Read the model definition and answer for the solid it produces. Units are mm, in the model's axes. Give positions to 0.01 mm unless a question says otherwise; leave off trailing zeros. Write each loop counter-clockwise with the first axis right and the second up, starting at its lowest first coordinate (ties: lowest second). Pieces come first, ordered by that corner, then holes. Notation, with made-up numbers: (-30, -32.75) -> (18, -32.75) arc R21 cw to (18, -15.75) -> close; hole circle Ø9 at (-38, 32.5). An arc over 180 degrees is marked (long way). Use a Markdown table: item, result.
from build123d import *

# Parameters (mm, degrees)
CROQUIS1_R              = 2
CROQUIS1_R_2            = 2.1
SALIENTE_EXTRUIR1_DEPTH = 2


with BuildPart() as part:
    # Croquis1 → Saliente-Extruir1 (new body)
    with BuildSketch(Plane(origin=(0, 0, 0), x_dir=(1, 0, 0), z_dir=(0, 1, 0))):
        with BuildLine():
            Line((-8, 5.5), (8, 5.5))
            ThreePointArc((8, 5.5), (11.5, 0), (8, -5.5))
            Line((8, -5.5), (-8, -5.5))
            ThreePointArc((-8, -5.5), (-11.5, 0), (-8, 5.5))
        make_face()
        with Locations(Location((8, 0, 0), (0, 0, 270))):
            Circle(CROQUIS1_R, mode=Mode.SUBTRACT)
        with Locations(Location((0, 0, 0), (0, 0, 270))):
            Circle(CROQUIS1_R_2, mode=Mode.SUBTRACT)
        with Locations(Location((-8, 0, 0), (0, 0, 270))):
            Circle(CROQUIS1_R, mode=Mode.SUBTRACT)
    extrude(amount=SALIENTE_EXTRUIR1_DEPTH)


solid = part.part
Item 1: Straight lines are drawn through the part: line 1 along X through (y, z) = (1.75, -1.25); line 2 along Z through (x, y) = (-0.5, 0.9); line 3 along Z through (x, y) = (-9, 0.6). For each, find the intervals that lie inside material, in ascending order. Write a range as [from, to].
Return value:
| item | result |
|---|---|
| line 1 | [-11.37, -9.56], [-6.44, -1.69], [1.69, 6.44], [9.56, 11.37] |
| line 2 | [-5.5, -2.04], [2.04, 5.5] |
| line 3 | [-4.91, -1.73], [1.73, 4.91] |
Item 2: A cutting plane is placed at C-C (z = -1). Give the vertices of the cut face in (x, y), then the cut area to 3 significant figures.
Return value:
| item | result |
|---|---|
| outline | (-11.42, 0) -> (-9.73, 0) -> (-9.73, 2) -> (-11.42, 2) -> close; (-6.27, 0) -> (-1.85, 0) -> (-1.85, 2) -> (-6.27, 2) -> close; (1.85, 0) -> (6.27, 0) -> (6.27, 2) -> (1.85, 2) -> close; (9.73, 0) -> (11.42, 0) -> (11.42, 2) -> (9.73, 2) -> close |
| area | 24.4 mm^2 |
Item 3: A cutting plane is placed at D-D (x = 7). Give the vertices of the cut face in (y, z).
Return value:
| item | result |
|---|---|
| outline | (0, -5.5) -> (2, -5.5) -> (2, -1.73) -> (0, -1.73) -> close; (0, 1.73) -> (2, 1.73) -> (2, 5.5) -> (0, 5.5) -> close |
Item 4: A cutting plane is placed at B-B (x = 0). Give the vertices of the cut face in (y, z).
Return value:
| item | result |
|---|---|
| outline | (0, -5.5) -> (2, -5.5) -> (2, -2.1) -> (0, -2.1) -> close; (0, 2.1) -> (2, 2.1) -> (2, 5.5) -> (0, 5.5) -> close |
Item 5: A cutting plane is placed at A-A (y = 1.2). Give the vertices of the cut face in (x, z).
Return value:
| item | result |
|---|---|
| outline | (-8, -5.5) -> (8, -5.5) arc R6.07 ccw to (8, 5.5) -> (-8, 5.5) arc R6.07 ccw to start; hole circle Ø4 at (-8, 0); hole circle Ø4.2 at (0, 0); hole circle Ø4 at (8, 0) |
Item 6: For a pull along X with two mould halves and no side action, classify faces 1 (the face through (0.631, 0.986, 2.003)), 2 (the face through (11.5, 1, -0.1)), 3 (the face through (0, 1, -5.5)) as +X half, -X half, draft (parallel to the pull), parting line (faces both ways), or undercut.
Return value:
| item | result |
|---|---|
| face 1 | undercut |
| face 2 | +X half |
| face 3 | draft |
